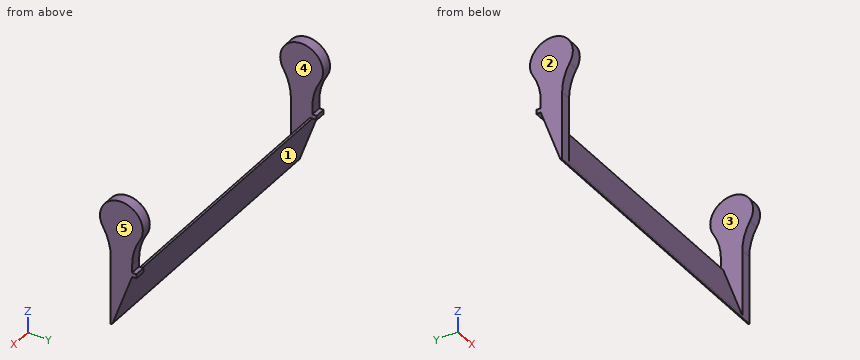
Autodesk Inventor part; units mm, degrees
ref_plane "Plano de trabajo1" through (67.5, 0, 0) normal (1, 0, 0) x (0, 0, -1)
ref_plane "YZ Plane" through (0, 0, 0) normal (1, 0, 0) x (0, 1, 0)
ref_plane "XZ Plane" through (0, 0, 0) normal (0, 1, 0) x (-1, 0, 0)
sketch "Boceto1" plane through (0, 0, 0) normal (1, 0, 0) x (0, 1, 0)
  arc A0 (8.5318, -5.2161) -> (-8.461, -5.3303) centre (0, 0) ccw
  line L0 (-5, -17.956) -> (-5, -50)
  line L1 (-5, -50) -> (-4.3301, -50)
  line L2 (5, -21.8397) -> (5, -18.1978)
  line L3 (0, 0) -> (8.6603, -5) construction
  line L4 (0, 0) -> (10, 0) construction
  line L5 (0, 0) -> (-8.6603, -5) construction
  line L6 (0, 0) -> (10, 0) construction
  arc A1 (8.6603, -5) -> (5, -18.1978) centre (30.624, -18.1978) ccw
  arc A2 (-5, -17.956) -> (-8.6603, -5) centre (-29.7601, -17.956) ccw
  line L7 (-4.3301, -50) -> (5, -23.8397)
  line L8 (5, -23.8397) -> (7, -23.8397)
  line L9 (7, -23.8397) -> (7, -21.8397)
  line L10 (7, -21.8397) -> (5, -21.8397)
  point P0 (-4.6651, -50)
  dimension "d3" = 30
  dimension "d4" = 210
  dimension "d8" = 50
  dimension "d16" = 10
extrude "Extrusión1" add sketch "Boceto1" along normal blind 5
sketch "Boceto3" plane through (5, 0, 0) normal (1, 0, 0) x (0, 0, -1)
  line L0 (23.8397, 5) -> (50, -4.3301)
  line L1 (23.8397, 3.9383) -> (48.9014, -5)
  line L2 (17.956, -5) -> (50, -5)
  line L3 (50, -4.3301) -> (50, -5)
  line L4 (48.9014, -5) -> (50, -5)
  line L5 (23.8397, 3.9383) -> (23.8397, 5)
  point P0 (0, 0)
  dimension "d12" = 1
extrude "Extrusión2" add sketch "Boceto3" along normal blind 125
ref_plane "Plano de trabajo1" through (67.5, 0, 0) normal (1, 0, 0) x (0, 0, -1)
mirror "Simetría1" about plane through (67.5, 0, 0) normal (1, 0, 0) of "Extrusión1"
fillet "Empalme1" radius 1 1 edges at (67.5, -4.3301, -50)
properties part number "cuchilla"
CAD build for the part. Positions are in the model's coordinates, mm. Face numbers are marked on the shaded views. A direction names the side the tool comes from. Coordinates: 2 decimals unless noted, no trailing zeros. Order: outer loops, then holes, each group sorted by start corner. A loop starts at its lowest first (then second) coordinate and runs counter-clockwise, first axis right, second up. Notation, with made-up numbers: M 1.5,56.25 L 53.5,56.25 A17 cw 53.5,69.25 Z; hole C 58.25,-18.75 d9. An arc over 180 degrees is marked long. Answer as CSV lines item,"result".
1) 3-axis set-ups, long thin cutter, end or side, ignore diameter. For the marked faces 4 and 5: which of +Z, -Z, +X, -X, +Y, -Y reach the whole face in a straight line?
Verdict:
face 4,"+Z, -Y"
face 5,"+Z, -Z, +X, +Y, -Y"
2) Cut at B-B (z = -7). List the corners of the cut face in (x, y), then the cut area to 3 significant figures.
Verdict:
outline,"M 0,-7.56 L 5,-7.56 L 5,7.58 L 0,7.58 Z; M 130,-7.56 L 135,-7.56 L 135,7.58 L 130,7.58 Z"
area,"151 mm2"
3) Mould opens along X. For the marked faces 1, 2 and 3 say: released by +X, released by -X, zero draft, split by the parting line, or undercut.
Verdict:
face 1,"zero draft"
face 2,"released by -X"
face 3,"undercut"
4) Cut at A-A (y = -6.75). List the corners of the cut face in (x, z).
Verdict:
outline,"M 0,-8.81 L 5,-8.81 L 5,7.38 L 0,7.38 Z; M 130,-8.81 L 135,-8.81 L 135,7.38 L 130,7.38 Z"
5) Cut at D-D (y = -0.25). List the corners of the cut face in (x, z).
Verdict:
outline,"M 0,-38.56 L 135,-38.56 L 135,10 L 130,10 L 130,-35.58 L 5,-35.58 L 5,10 L 0,10 Z"
6) Flat gauge pins, fed straight in: P1, Ø1.6, axis at x = 1.5, z = -22.5, coming from the +Y side; P2, Ø4, axis at x = 2.5, z = -19, coming from the +Y side; P3, Ø9.5, axis at x = 94.5, z = -31, coming from the -Y side; P4, Ø10, axis at y = 2.5, z = -28, coming from the -X side. Where does each tip first touch, or does it go through?
Verdict:
P1,"y = 7"
P2,"y = 5.03"
P3,"y = -0.31"
P4,"x = 0"
7) Drill centre lines: L1, parallel to X at y = -7.25, z = -4; L2, parallel to Y at x = 17.5, z = -33; L3, parallel to Y at x = 51, z = -40. Where is each one in solid material? Low to high. Write a range as from..to.
Verdict:
L1,"0..5, 130..135"
L2,"0.67..1.73"
L3,"-1.83..-0.76"
8) Cut at C-C (x = 85). List the corners of the cut face in (y, z), then the cut area to 3 significant figures.
Verdict:
outline,"M -5,-50 A1 ccw -4.09,-49.34 L 5,-23.84 L 3.94,-23.84 L -5,-48.9 Z"
area,"27.5 mm2"
